For this review, take the finished solid that the model builds, in its own axes (mm). A direction names the side the tool comes from. Give positions to 0.01 mm unless a question says otherwise; leave off trailing zeros. Write each loop counter-clockwise with the first axis right and the second up, starting at its lowest first coordinate (ties: lowest second). Pieces come first, ordered by that corner, then holes. Notation, with made-up numbers: (49.25, -5) -> (85.25, -5) arc R16 cw to (85.25, 11) -> close; hole circle Ø11 at (70.5, 62.5). An arc over 180 degrees is marked (long way). Answer as CSV lines item,"result".
```python
from build123d import *

# Parameters (mm, degrees)
SKICA1_W                    = 35
SKICA1_H                    = 60
P_IDAT_VYSUNUT_M1_DEPTH     = 3
SKICA3_W                    = 45
SKICA3_H                    = 70
SKICA3_W_2                  = 35
SKICA3_H_2                  = 60
VYSUNOUT_TENKOST_NN_1_DEPTH = 20
SKICA4_R                    = 3.75
SKICA4_R_2                  = 1.75
VYSUNOUT_TENKOST_NN_2_DEPTH = 2
ODEBRAT_START               = -1.5
SKICA5_R                    = 1.75
ODEBRAT_VYSUNUT_M1_DEPTH    = 1.5
SKICA10_W                   = 45
SKICA10_H                   = 70
P_IDAT_VYSUNUT_M2_DEPTH     = 5
SKICA12_W                   = 35
SKICA12_H                   = 50.840130339
ODEBRAT_VYSUNUT_M5_DEPTH    = 5
SKICA13_W                   = 45
SKICA13_H                   = 70
P_IDAT_VYSUNUT_M3_DEPTH     = 5
P_IDAT_VYSUNUT_M5_DEPTH     = 50
SKICA17_W                   = 45
SKICA17_H                   = 70
P_IDAT_VYSUNUT_M6_DEPTH     = 5
SKICA7_R                    = 2
ODEBRAT_VYSUNUT_M3_DEPTH    = 3.2
ODEBRAT_VYSUNUT_M6_REACH    = 104.22
SKICA8_W                    = 10
SKICA8_H                    = 4
SKICA21_W                   = 60
SKICA21_H                   = 70
ODEBRAT_VYSUNUT_M7_DEPTH    = 3
SKICA22_R                   = 1.75
ODEBRAT_VYSUNUT_M8_DEPTH    = 5
SKICA23_R                   = 5
ODEBRAT_VYSUNUT_M9_DEPTH    = 5


with BuildPart() as part:
    # Skica1 → Přidat vysunutím1 (new body)
    with BuildSketch(Plane.XY):
        with Locations((17.5, 30)):
            Rectangle(SKICA1_W, SKICA1_H)
    extrude(amount=P_IDAT_VYSUNUT_M1_DEPTH)

    # Skica3 → Vysunout tenkostěnný1 (add)
    with BuildSketch(Plane(origin=(0, 0, 0), x_dir=(-1, 0, 0), z_dir=(0, 0, -1))):
        with Locations((-17.5, 30)):
            Rectangle(SKICA3_W, SKICA3_H)
        with Locations((-17.5, 30)):
            Rectangle(SKICA3_W_2, SKICA3_H_2, mode=Mode.SUBTRACT)
    extrude(amount=-VYSUNOUT_TENKOST_NN_1_DEPTH)

    # Skica4 → Vysunout tenkostěnný2 (add)
    # profile 1 of 4: a face of its own
    with BuildSketch(Plane.XY.offset(3)):
        with Locations((4, 55)):
            Circle(SKICA4_R)
        with Locations((4, 55)):
            Circle(SKICA4_R_2, mode=Mode.SUBTRACT)
    # profile 2 of 4: a face of its own
    with BuildSketch(Plane.XY.offset(3)):
        with Locations((31, 55)):
            Circle(SKICA4_R)
        with Locations((31, 55)):
            Circle(SKICA4_R_2, mode=Mode.SUBTRACT)
    # profile 3 of 4: a face of its own
    with BuildSketch(Plane.XY.offset(3)):
        with Locations((31, 10)):
            Circle(SKICA4_R)
        with Locations((31, 10)):
            Circle(SKICA4_R_2, mode=Mode.SUBTRACT)
    # profile 4 of 4: a face of its own
    with BuildSketch(Plane.XY.offset(3)):
        with Locations((4, 10)):
            Circle(SKICA4_R)
        with Locations((4, 10)):
            Circle(SKICA4_R_2, mode=Mode.SUBTRACT)
    extrude(amount=VYSUNOUT_TENKOST_NN_2_DEPTH)

    # Skica5 → Odebrat vysunutím1 (cut)
    with BuildSketch(Plane.XY.offset(3).offset(ODEBRAT_START)):
        with Locations((4, 55)):
            Circle(SKICA5_R)
        with Locations((31, 55)):
            Circle(SKICA5_R)
        with Locations((31, 10)):
            Circle(SKICA5_R)
        with Locations((4, 10)):
            Circle(SKICA5_R)
    extrude(amount=ODEBRAT_VYSUNUT_M1_DEPTH, mode=Mode.SUBTRACT)

    # Skica10 → Přidat vysunutím2 (add)
    with BuildSketch(Plane(origin=(0, 0, 0), x_dir=(-1, 0, 0), z_dir=(0, 0, -1))):
        with Locations((-17.5, 30)):
            Rectangle(SKICA10_W, SKICA10_H)
    extrude(amount=P_IDAT_VYSUNUT_M2_DEPTH)

    # Skica12 → Odebrat vysunutím5 (cut)
    with BuildSketch(Plane(origin=(0, 0, -5), x_dir=(-1, 0, 0), z_dir=(0, 0, -1))):
        with Locations((-17.5, 39.579934831)):
            Rectangle(SKICA12_W, SKICA12_H)
    extrude(amount=-ODEBRAT_VYSUNUT_M5_DEPTH, mode=Mode.SUBTRACT)

    # Skica13 → Přidat vysunutím3 (add)
    with BuildSketch(Plane(origin=(0, 0, -5), x_dir=(-1, 0, 0), z_dir=(0, 0, -1))):
        with Locations((-17.5, 30)):
            Rectangle(SKICA13_W, SKICA13_H)
    extrude(amount=P_IDAT_VYSUNUT_M3_DEPTH)

    # Skica16 → Přidat vysunutím5 (add)
    with BuildSketch(Plane(origin=(0, 0, -10), x_dir=(-1, 0, 0), z_dir=(0, 0, -1))):
        Polygon((-37, -5), (5, -5), (5, 0), (-35, 0), (-35, 60), (5, 60), (5, 65), (-37, 65), (-40, 65), (-40, 62), (-40, -2), (-40, -5), align=None)
    extrude(amount=P_IDAT_VYSUNUT_M5_DEPTH)

    # Skica17 → Přidat vysunutím6 (add)
    with BuildSketch(Plane(origin=(0, 0, -60), x_dir=(-1, 0, 0), z_dir=(0, 0, -1))):
        with Locations((-17.5, 30)):
            Rectangle(SKICA17_W, SKICA17_H)
    extrude(amount=P_IDAT_VYSUNUT_M6_DEPTH)

    # Skica7 → Odebrat vysunutím3 (cut)
    with BuildSketch(Plane.XY.offset(20)):
        with Locations((37, 62)):
            Circle(SKICA7_R)
        with Locations((-2, 62)):
            Circle(SKICA7_R)
        with Locations((-2, -2)):
            Circle(SKICA7_R)
        with Locations((37, -2)):
            Circle(SKICA7_R)
    extrude(amount=-ODEBRAT_VYSUNUT_M3_DEPTH, mode=Mode.SUBTRACT)

    # Skica8 → Odebrat vysunutím6 (cut, up to next)
    with BuildSketch(Plane.XY.offset(3), mode=Mode.PRIVATE) as odebrat_vysunut_m6_sk1:
        with Locations((17.5, 3)):
            Rectangle(SKICA8_W, SKICA8_H)
    odebrat_vysunut_m6_tool1 = extrude(odebrat_vysunut_m6_sk1.sketch, amount=-ODEBRAT_VYSUNUT_M6_REACH, mode=Mode.PRIVATE) & part.part
    add(odebrat_vysunut_m6_tool1.solids().sort_by_distance((17.5, 3, 3))[0], mode=Mode.SUBTRACT)

    # Skica21 → Odebrat vysunutím7 (cut)
    with BuildSketch(Plane.ZY.offset(5)):
        with Locations((-35, 30)):
            Rectangle(SKICA21_W, SKICA21_H)
    extrude(amount=-ODEBRAT_VYSUNUT_M7_DEPTH, mode=Mode.SUBTRACT)

    # Skica22 → Odebrat vysunutím8 (cut)
    with BuildSketch(Plane.ZY.offset(2)):
        with Locations((-7.5, 62.5)):
            Circle(SKICA22_R)
        with Locations((-7.5, -2.5)):
            Circle(SKICA22_R)
        with Locations((-62.5, -2.5)):
            Circle(SKICA22_R)
        with Locations((-62.5, 62.5)):
            Circle(SKICA22_R)
    extrude(amount=-ODEBRAT_VYSUNUT_M8_DEPTH, mode=Mode.SUBTRACT)

    # Skica23 → Odebrat vysunutím9 (cut)
    with BuildSketch(Plane.XZ.offset(5)):
        with Locations(Location((14.5, -45.923378455, 0), (0, 0, 270))):
            Circle(SKICA23_R)
    extrude(amount=-ODEBRAT_VYSUNUT_M9_DEPTH, mode=Mode.SUBTRACT)


solid = part.part
```
Q1. Add section D-D (z = -7.5). Write out the cut boundary in (x, y), plus the area to 4 significant figures.
Answer block:
outline,"(-2, -5) -> (40, -5) -> (40, 65) -> (-2, 65) -> (-2, 64.25) -> (3, 64.25) -> (3, 60.75) -> (-2, 60.75) -> (-2, -0.75) -> (3, -0.75) -> (3, -4.25) -> (-2, -4.25) -> close; hole (12.5, 1) -> (22.5, 1) -> (22.5, 5) -> (12.5, 5) -> close"
area,"2,865 mm2"
Q2. Add section B-B (x = 14.5). Write out the cut boundary in (y, z).
Answer block:
outline,"(-5, -65) -> (65, -65) -> (65, -5) -> (14.16, -5) -> (14.16, 0) -> (65, 0) -> (65, 20) -> (60, 20) -> (60, 3) -> (5, 3) -> (5, -10) -> (60, -10) -> (60, -60) -> (0, -60) -> (0, -50.92) -> (-5, -50.92) -> close; (-5, -40.92) -> (0, -40.92) -> (0, -10) -> (1, -10) -> (1, 3) -> (0, 3) -> (0, 20) -> (-5, 20) -> close"
Q3. To check wall thickness, follow probe 1 along Z at (x, y) = (26, 26.5); probe 2 along Y at (x, z) = (4, 2); probe 3 along Z at (x, y) = (11.5, 5). State the ranges of each line that lie inside material, in increasing order. Write a range as [from, to].
Answer block:
probe 1,"z = [-65, -60], [-10, -5], [0, 3]"
probe 2,"y = [-5, 8.25], [11.75, 53.25], [56.75, 65]"
probe 3,"z = [-65, -60], [-10, 3]"
Q4. For faces 1 (the flat face through (17, 30, 3)), 2 (the flat face through (3, 63, -63)), list the 3-axis set-ups (+Z, -Z, +X, -X, +Y, -Y) from which the entire face can be reached by the end or side of a thin tool; tool diameter is ignored.
Answer block:
face 1,"+Z"
face 2,"-X"
Q5. Clearance check with flat-ended pins moving along their axes: pin 1 (4 mm diameter, centred on x = 3.5, y = 10, fed in from +Z); pin 2 (3 mm diameter, centred on x = 30.5, y = 37, fed in from +Z); pin 3 (6 mm diameter, centred on x = 14.5, z = -45.92, fed in from -Y). State where each tip first meets the part, or that it passes through.
Answer block:
pin 1,"stops at z = 5"
pin 2,"stops at z = 3"
pin 3,"stops at y = 60"
Q6. Draft analysis for pull direction Z (two halves, no side actions). For faces 3 (the cylindrical face through (0.465, 61.83, -60.883)), 4 (the flat face through (4, 10, 1.5)), 5 (the cylindrical face through (3.62, 53.29, 3.23)), state which applies: released by +Z, released by -Z, zero draft, split by the parting line, or undercut.
Answer block:
face 3,"undercut"
face 4,"released by +Z"
face 5,"zero draft"
